Build history of the part. All positions in model axes, mm. Face numbers are marked on the shaded views. A direction names the side the tool comes from. Give positions to 0.01 mm unless a question says otherwise; leave off trailing zeros. Write each loop counter-clockwise with the first axis right and the second up, starting at its lowest first coordinate (ties: lowest second). Pieces come first, ordered by that corner, then holes.
from build123d import *

# Parameters (mm, degrees)
F1_DEPTH    = 77.978
F2_R        = 9.8113639175
F3_T1_DEPTH = 141.3502926448
F4_SIZE     = 5.08


# Not quite as in the source:
# - a fillet or chamfer that OpenCascade refuses, or shapes differently, is made with other operations: its cross-section is extruded or revolved along the edge and cut away or added


with BuildPart() as f1:
    # F0 (on Top) → F1 (new body)
    with BuildSketch(Plane.XY):
        with BuildLine():
            Line((-7.4381157756, 43.2214848697), (-39.8039706051, 38.5977886617))
            ThreePointArc((-39.8039706051, 38.5977886617), (-21.172854192, -38.7924441896), (19.2988961935, 29.7524612397))
            Line((19.2988961935, 29.7524612397), (-14.8171193926, 3.6754181444))
            Line((-14.8171193926, 3.6754181444), (-26.3349507004, 16.8865323067))
            ThreePointArc((-26.3349507004, 16.8865323067), (-4.9953492686, 21.5214038686), (-7.4381157756, 43.2214848697))
        make_face()
    extrude(amount=F1_DEPTH)

    # F2
    f2_edges = [f1.edges().sort_by_distance(p)[0] for p in [
        (19.298896, 29.752461, 38.989),
    ]]
    fillet(f2_edges, radius=F2_R)

    # F3: chamfer of 5.08 on 1 edges, made by hand

    # F3_s2 → F3_t1 (cut)
    with BuildSketch(Plane.XY.offset(-31.6861463224)):
        with BuildLine():
            Line((-14.6495810062, 42.3422516773), (-1.8120830861, 31.8641235926))
            Line((-1.8120830861, 31.8641235926), (-1.7106647042, 31.8701958104))
            ThreePointArc((-1.7106647042, 31.8701958104), (-3.4500397911, 38.1062153929), (-7.3708029252, 43.2975870391))
            Line((-7.3708029252, 43.2975870391), (-7.4524841935, 43.3220637371))
            ThreePointArc((-7.4524841935, 43.3220637371), (-11.0476484326, 42.8084685502), (-14.663949424, 42.4428305447))
            Line((-14.663949424, 42.4428305447), (-14.6495810062, 42.3422516773))
        make_face()
    extrude(amount=F3_T1_DEPTH, mode=Mode.SUBTRACT)

    # F4
    f4_edges = [f1.edges().sort_by_distance(p)[0] for p in [
        (-27.46138, -37.361606, 77.978),
        (19.021994, 24.517514, 77.978),
        (-2.246992, 13.283567, 77.978),
    ]]
    chamfer(f4_edges, length=F4_SIZE)


solid = f1.part
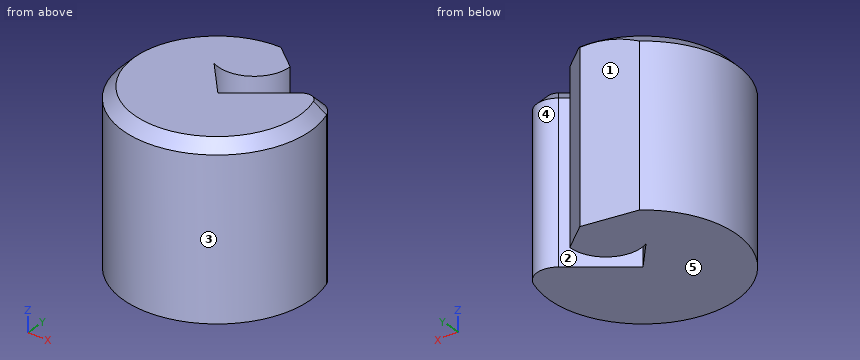
(1) 3-axis set-ups, long thin cutter, end or side, ignore diameter. For the marked faces 1 and 2: which of +Z, -Z, +X, -X, +Y, -Y reach the whole face in a straight line?
(2) Drop flat-ended pins along their axis: pin 1 (2 mm diameter, centred on x = 4, z = 53, fed in from +Y); pin 2 (6 mm diameter, centred on x = -29.5, z = 42, fed in from -Y); pin 3 (12 mm diameter, centred on y = -18.5, z = 13.5, fed in from -X). Give the stop position or say it passes through.
(3) Mould opens along X. For the marked faces 3, 4 and 5 say: +X half, -X half, draft (parallel to the pull), parting line (faces both ways), or undercut.
(4) Probe line 1 (Y direction, x = -4.5, z = 9.5); line 2 (Y direction, x = -12, z = 17.5); line 3 (X direction, y = 21, z = 22.5). List the from-to ranges inside material, lowest first.
(5) Saw through at A-A, the plane z = 65. List the corners of the cut face in (x, y).
Computed values:
1. face 1: +Z, -Z, -X, +Y
1. face 2: +Z, -Z
2. pin 1: stops at y = 18.82
2. pin 2: stops at y = -37.65
2. pin 3: stops at x = -54.59
3. face 3: parting line
3. face 4: undercut
3. face 5: draft
4. line 1: y = -38.01 to 11.56, 22.25 to 34.06
4. line 2: y = -39.17 to 5.83, 15.97 to 40.18
4. line 3: x = -54.11 to -5.39, 7.85 to 24.12
5. outline: (-39.8, 38.6) arc R42.94 ccw (long way) to (25.49, 18.48) arc R9.81 ccw to (10.32, 22.89) - (-14.82, 3.68) - (-26.33, 16.89) arc R16.29 ccw to (-1.97, 31.99) - (-14.49, 42.21) - close
